Could you check a few things on this model? Use its own coordinates, in mm. Coordinates: 2 decimals unless noted, no trailing zeros. Loops run counter-clockwise (first coordinate to the right, second up) from the corner with the lowest first, then second, coordinate; pieces in that order, holes last. Notation, with made-up numbers: M -21,5 L 2,5 A17 cw 2,34 Z; hole C -29.75,21 d10. An arc over 180 degrees is marked long. Use one line per item in the form item = value. Start each with the question number.
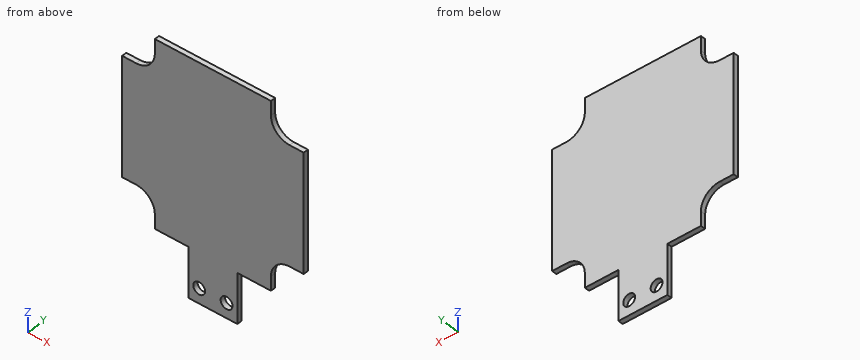
```python
from build123d import *

# Parameters (mm, degrees)
BOSS_EXTRUDE1_DEPTH = 1.4
SKETCH2_R           = 1.25
CUT_EXTRUDE2_DEPTH  = 48.727979216
CUT_EXTRUDE3_DEPTH  = 48.727979216
SKETCH6_R           = 1.7
CUT_EXTRUDE4_DEPTH  = 48.727979216


with BuildPart() as part:
    # Sketch1 → Boss-Extrude1 (new body)
    with BuildSketch(Plane(origin=(0, 0, 0), x_dir=(1, 0, 0), z_dir=(0, 1, 0))):
        Polygon((26, -26), (-26, -26), (-26, 26), (-7, 26), (-7, 40), (7, 40), (7, 26), (26, 26), align=None)
    extrude(amount=BOSS_EXTRUDE1_DEPTH)

    # Sketch2 → Cut-Extrude2 (cut, through all)
    with BuildSketch(Plane(origin=(0, 0, 0), x_dir=(1, 0, 0), z_dir=(0, 1, 0))):
        with Locations(Location((-22, 22, 0), (0, 0, 270))):
            Circle(SKETCH2_R)
        with Locations(Location((22, 22, 0), (0, 0, 90))):
            Circle(SKETCH2_R)
        with Locations(Location((22, -22, 0), (0, 0, 270))):
            Circle(SKETCH2_R)
        with Locations(Location((-22, -22, 0), (0, 0, 90))):
            Circle(SKETCH2_R)
    extrude(amount=CUT_EXTRUDE2_DEPTH, mode=Mode.SUBTRACT)

    # Sketch5 → Cut-Extrude3 (cut, through all)
    with BuildSketch(Plane(origin=(0, 1.4, 0), x_dir=(1, 0, 0), z_dir=(0, 1, 0))):
        with BuildLine():
            Line((-26, 26), (-16.625, 26))
            Line((-16.625, 26), (-16.625, 22))
            ThreePointArc((-16.625, 22), (-18.199301051, 18.199301051), (-22, 16.625))
            Line((-22, 16.625), (-26, 16.625))
            Line((-26, 16.625), (-26, 26))
        make_face()
        with BuildLine():
            Line((22, 16.625), (26, 16.625))
            Line((26, 16.625), (26, 26))
            Line((26, 26), (16.625, 26))
            Line((16.625, 26), (16.625, 22))
            ThreePointArc((16.625, 22), (18.199301051, 18.199301051), (22, 16.625))
        make_face()
        with BuildLine():
            Line((-22, -16.625), (-26, -16.625))
            Line((-26, -16.625), (-26, -26))
            Line((-26, -26), (-16.625, -26))
            Line((-16.625, -26), (-16.625, -22))
            ThreePointArc((-16.625, -22), (-18.199301051, -18.199301051), (-22, -16.625))
        make_face()
        with BuildLine():
            Line((26, -26), (16.625, -26))
            Line((16.625, -26), (16.625, -22))
            ThreePointArc((16.625, -22), (18.199301051, -18.199301051), (22, -16.625))
            Line((22, -16.625), (26, -16.625))
            Line((26, -16.625), (26, -26))
        make_face()
    extrude(amount=-CUT_EXTRUDE3_DEPTH, mode=Mode.SUBTRACT)

    # Sketch6 → Cut-Extrude4 (cut, through all)
    with BuildSketch(Plane(origin=(0, 1.4, 0), x_dir=(1, 0, 0), z_dir=(0, 1, 0))):
        with Locations(Location((3.925, 35.8, 0), (0, 0, 270))):
            Circle(SKETCH6_R)
        with Locations(Location((-3.925, 35.8, 0), (0, 0, 270))):
            Circle(SKETCH6_R)
    extrude(amount=-CUT_EXTRUDE4_DEPTH, mode=Mode.SUBTRACT)


solid = part.part
```
Item 1: I want a section at B-B (y = 1). Write out the boundary of the cut face in (x, z) (3 decimals).
Item 2: Please list where these lines run through material, in increasing order: line 1 along X through (y, z) = (0.6, -35.8) (3 decimals); line 2 along X through (y, z) = (0.2, 22) (3 decimals); line 3 along X through (y, z) = (0.5, -36.5).
Item 3: I'm going to push flat-ended pins straight in: P1, Ø0.7, axis at y = 0.5, z = -23.5, coming from the +X side (3 decimals); P2, Ø0.7, axis at x = -11.5, y = 0.5, coming from the -Z side; P3, Ø2, axis at x = 3.925, z = -35.8, coming from the +Y side. Where does each tip first touch, or does it pass through?
Item 4: I want a section at D-D (z = -21). Write out the boundary of the cut face in (x, y), plus the area to 3 significant figures.
Item 5: I want a section at A-A (z = -35.8). Write out the boundary of the cut face in (x, y) (3 decimals), plus the area to 3 significant figures.
Item 6: I want a section at C-C (x = -10.5). Write out the boundary of the cut face in (y, z).
Worked answers:
q1.outline = M -26,-16.625 L -22,-16.625 A5.375 cw -16.625,-22 L -16.625,-26 L -7,-26 L -7,-40 L 7,-40 L 7,-26 L 16.625,-26 L 16.625,-22 A5.375 cw 22,-16.625 L 26,-16.625 L 26,16.625 L 22,16.625 A5.375 cw 16.625,22 L 16.625,26 L -16.625,26 L -16.625,22 A5.375 cw -22,16.625 L -26,16.625 Z; hole C -3.925,-35.8 d3.4; hole C 3.925,-35.8 d3.4
q2.line_1 = -7 to -5.625, -2.225 to 2.225, 5.625 to 7
q2.line_2 = -16.625 to 16.625
q2.line_3 = -7 to -5.47, -2.38 to 2.38, 5.47 to 7
q3.P1 = 16.625
q3.P2 = -26
q3.P3 = through
q4.outline = M -16.72,0 L 16.72,0 L 16.72,1.4 L -16.72,1.4 Z
q4.area = 46.8 mm²
q5.outline = M -7,0 L -5.625,0 L -5.625,1.4 L -7,1.4 Z; M -2.225,0 L 2.225,0 L 2.225,1.4 L -2.225,1.4 Z; M 5.625,0 L 7,0 L 7,1.4 L 5.625,1.4 Z
q5.area = 10.1 mm²
q6.outline = M 0,-26 L 1.4,-26 L 1.4,26 L 0,26 Z
